```python
from build123d import *

# Parameters (mm, degrees)
F0_R     = 19.35
F1_DEPTH = 25
F4_R     = 14.671032
F4_R_2   = 10.237718
F5_DEPTH = 26.6


with BuildPart() as f1:
    # F0 (on Top) → F1 (new body)
    with BuildSketch(Plane.XY):
        Circle(F0_R)
    extrude(amount=F1_DEPTH)

    # F2 (on Right) → F3 (revolve)
    with BuildSketch(Plane.YZ):
        Polygon((0, 24.767736), (19.990396, 24.767736), (0, 74.592263), align=None)
    revolve(axis=Axis((0, 0, 4.910189), (0, 0, 1)))

    # F4 (on Top) → F5 (join)
    with BuildSketch(Plane.XY):
        Circle(F4_R)
        Circle(F4_R_2, mode=Mode.SUBTRACT)
    extrude(amount=-F5_DEPTH)


solid = f1.part
```
Build history of the part. All positions in model axes, mm. A direction names the side the tool comes from. Round coordinates to 2 decimals unless told otherwise and drop trailing zeros. Order: outer loops, then holes, each group sorted by start corner. A loop starts at its lowest first (then second) coordinate and runs counter-clockwise, first axis right, second up. Notation, with made-up numbers: (52, 15) -> (72, 15) arc R24 cw to (72, 36) -> close; hole circle Ø11 at (10.25, 41.25). An arc over 180 degrees is marked (long way). Answer in a Markdown table with one row per item.
1) Band-saw the part on A-A on z = -6.5. Give the cut face in (x, y), and give its area (3 significant figures).
Values:
| item | result |
|---|---|
| outline | circle Ø29.34 at (0, 0); hole circle Ø20.48 at (0, 0) |
| area | 347 mm2 |
2) Band-saw the part on B-B on z = 58.5. Give the cut face in (x, y), and give its area (3 significant figures).
Values:
| item | result |
|---|---|
| outline | circle Ø12.91 at (0, 0) |
| area | 131 mm2 |
3) Pin check, flat tips, straight feed: P1, Ø1, axis at y = 13, z = 29, coming from the +X side; P2, Ø16.5, axis at x = 0, y = 0, coming from the -Z side; P3, Ø6, axis at x = 6, y = -8.5, coming from the +Z side. Stop position of each tip, or through.
Values:
| item | result |
|---|---|
| P1 | x = 13.43 |
| P2 | z = 0 |
| P3 | z = 56.14 |
4) Wall check: L1, parallel to Y at x = 0, z = -5; L2, parallel to Y at x = 9, z = -13.5; L3, parallel to X at y = 2, z = -6.5. Give the ranges that are in metal, low to high.
Values:
| item | result |
|---|---|
| L1 | -14.67 to -10.24, 10.24 to 14.67 |
| L2 | -11.59 to -4.88, 4.88 to 11.59 |
| L3 | -14.53 to -10.04, 10.04 to 14.53 |
5) Which spindle directions (+Z, -Z, +X, -X, +Y, -Y) get a long thin tool onto all of the face, cutting with end or side? Do faces 1 (the flat face through (3, 10, -26.6)), 2 (the cylindrical face through (-19.33, 0.85, 12.21)). Say none if no direction does.
Values:
| item | result |
|---|---|
| face 1 | -Z, +X, -X, +Y, -Y |
| face 2 | -Z |
6) Mould opens along Y. For faces 3 (the cylindrical face through (-8.124, -6.229, -13.114)), 4 (the conical face through (-2.293, 7.282, 55.565)), 5 (the flat face through (0, 0, 0)), 6 (the flat face through (-14.4, 4.4, 0)) say: released by +Y, released by -Y, zero draft, split by the parting line, or undercut.
Values:
| item | result |
|---|---|
| face 3 | undercut |
| face 4 | split by the parting line |
| face 5 | undercut |
| face 6 | zero draft |
